```python
from build123d import *

# Parameters (mm, degrees)
SKETCH1_W           = 10
SKETCH1_H           = 10.813
BOSS_EXTRUDE1_DEPTH = 2
SKETCH2_W           = 10
SKETCH2_H           = 2.5
BOSS_EXTRUDE2_DEPTH = 5
SKETCH3_R           = 1
CUT_EXTRUDE1_DEPTH  = 11.813
FILLET2_R           = 2


with BuildPart() as part:
    # Sketch1 → Boss-Extrude1 (new body)
    with BuildSketch(Plane.XY):
        with Locations((-3.333333333, -1.47534058)):
            Rectangle(SKETCH1_W, SKETCH1_H)
    extrude(amount=BOSS_EXTRUDE1_DEPTH)

    # Sketch2 → Boss-Extrude2 (add)
    with BuildSketch(Plane.XY.offset(2)):
        with Locations((-3.333333333, 2.68115942)):
            Rectangle(SKETCH2_W, SKETCH2_H)
        with Locations((-3.333333333, -5.63184058)):
            Rectangle(SKETCH2_W, SKETCH2_H)
    extrude(amount=BOSS_EXTRUDE2_DEPTH)

    # Sketch3 → Cut-Extrude1 (cut, through all)
    with BuildSketch(Plane(origin=(0, 3.93115942, 0), x_dir=(1, 0, 0), z_dir=(0, 1, 0))):
        with Locations((-3.318584334, -4.43)):
            Circle(SKETCH3_R)
    extrude(amount=-CUT_EXTRUDE1_DEPTH, mode=Mode.SUBTRACT)

    # Fillet2
    fillet2_edges = [part.edges().sort_by_distance(p)[0] for p in [
        (-8.333333333, 2.68115942, 7),
        (1.666666667, 2.68115942, 7),
        (1.666666667, -5.63184058, 7),
        (-8.333333333, -5.63184058, 7),
        (-3.333333333, 3.93115942, 0),
        (-3.333333333, -6.88184058, 0),
    ]]
    fillet(fillet2_edges, radius=FILLET2_R)


solid = part.part
```
Verification items for the finished model (mm, model axes). A direction names the side the tool comes from. Coordinates: 2 decimals unless noted, no trailing zeros. Loops run counter-clockwise (first coordinate to the right, second up) from the corner with the lowest first, then second, coordinate; pieces in that order, holes last. Notation, with made-up numbers: (85, 40) - (115, 40) arc R14 ccw to (115, 57) - close; hole circle Ø2 at (-27, 1). An arc over 180 degrees is marked (long way). Put each result on its own line as item: value.
Item 1: Set-up check for faces 1 (the face through (-3, -1, 0)), 2 (the face through (-3, 1.431, 3)): record each of +Z, -Z, +X, -X, +Y, -Y from which the full face is reachable in a straight line by a thin tool's end or side.
Conclusion:
face 1: -Z, +X, -X, +Y, -Y
face 2: +Z, +X, -X
Item 2: Section check C-C (z = 4.43). Enter the section's corners in (x, y), then the cut area to 3 significant figures.
Conclusion:
outline: (-8.33, -6.88) - (-4.32, -6.88) - (-4.32, -4.38) - (-8.33, -4.38) - close; (-8.33, 1.43) - (-4.32, 1.43) - (-4.32, 3.93) - (-8.33, 3.93) - close; (-2.32, -6.88) - (1.67, -6.88) - (1.67, -4.38) - (-2.32, -4.38) - close; (-2.32, 1.43) - (1.67, 1.43) - (1.67, 3.93) - (-2.32, 3.93) - close
area: 40.0 mm2
Item 3: Section check D-D (y = -5.75). Enter the section's corners in (x, z), then the cut area to 3 significant figures.
Conclusion:
outline: (-8.33, 0.2) - (1.67, 0.2) - (1.67, 5) arc R2 ccw to (-0.33, 7) - (-6.33, 7) arc R2 ccw to (-8.33, 5) - close; hole circle Ø2 at (-3.32, 4.43)
area: 63.2 mm2
Item 4: Gauge pin test, flat end, axial feed: pin 1 Ø1 at (x, y) = (-4, -0.5) entering from +Z. Record the tip position at first contact, or that the pin passes through.
Conclusion:
pin 1: stops at z = 2
Item 5: Draft check along Y on faces 3 (the face through (-3, -4.382, 3)), 4 (the face through (-3, -1, 2)), 5 (the face through (-3.26, -6.28, 0.57)), 6 (the face through (1.065, 2.699, 6.43)). Enter one of: pulls with the +Y half, pulls with the -Y half, needs draft (parallel to the pull), parting line crosses it, or undercut.
Conclusion:
face 3: undercut
face 4: undercut
face 5: pulls with the -Y half
face 6: needs draft
Item 6: Section check A-A (z = 2.75). Enter the section's corners in (x, y), then the cut area to 3 significant figures.
Conclusion:
outline: (-8.33, -6.88) - (1.67, -6.88) - (1.67, -4.38) - (-8.33, -4.38) - close; (-8.33, 1.43) - (1.67, 1.43) - (1.67, 3.93) - (-8.33, 3.93) - close
area: 50.0 mm2
Item 7: Section check B-B (x = -1.5). Enter the section's corners in (y, z), then the cut area to 3 significant figures.
Conclusion:
outline: (-6.88, 2) arc R2 ccw to (-4.88, 0) - (1.93, 0) arc R2 ccw to (3.93, 2) - (3.93, 7) - (1.43, 7) - (1.43, 2) - (-4.38, 2) - (-4.38, 7) - (-6.88, 7) - close
area: 44.9 mm2
Item 8: Scan lines: line 1 along X through (y, z) = (2.7, 4.43); line 2 along Y through (x, z) = (-7, 4.5); line 3 along Z through (x, y) = (-7, -0.5). Record each from-to range of solid material in increasing order.
Conclusion:
line 1: x = -8.33 to -4.32, -2.32 to 1.67
line 2: y = -6.88 to -4.38, 1.43 to 3.93
line 3: z = 0 to 2
